Check sheet for the modelled part. Datum: model origin and axes. Units: mm. Round coordinates to 2 decimals unless told otherwise and drop trailing zeros. Loops run counter-clockwise (first coordinate to the right, second up) from the corner with the lowest first, then second, coordinate; pieces in that order, holes last. Notation, with made-up numbers: (67, -18) - (98, -18) arc R33 ccw to (98, 13) - close; hole circle Ø1 at (19, 59). An arc over 180 degrees is marked (long way). Answer in a Markdown table with one row per item. Add a question column.
(1) Cross-section at A-A on z = -84. Enter the section's corners in (x, y), then the cut area to 3 significant figures.
(2) Thickness scan on line 1 along Y through (x, z) = (0, -12); line 2 along X through (y, z) = (23, -155.5); line 3 along Y through (x, z) = (326, -58.5). Record the ranges inside material, lowest first.
(3) Gauge pin test, flat ends, axial feed: pin 1 (12 mm diameter, centred on x = -119.5, y = 486, fed in from +Z); pin 2 (3 mm diameter, centred on x = -34.5, y = -123.5, fed in from +Z); pin 3 (3 mm diameter, centred on y = -103, z = -74, fed in from +X). Record the tip position at first contact, or that the pin passes through.
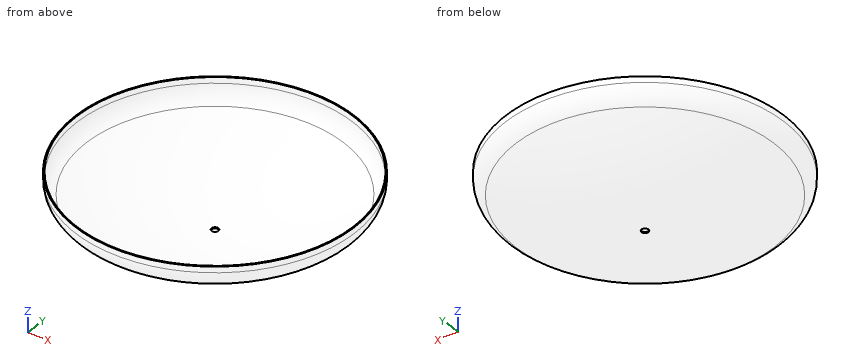
Autodesk Inventor part; units mm, degrees
ref_plane "YZ Plane" through (0, 0, 0) normal (1, 0, 0) x (0, 1, 0)
ref_plane "XZ Plane" through (0, 0, 0) normal (0, 1, 0) x (-1, 0, 0)
ref_plane "XY Plane" through (0, 0, 0) normal (0, 0, 1) x (1, 0, 0)
sketch "Sketch1" plane through (0, 0, 0) normal (0, 1, 0) x (-1, 0, 0)
  line L0 (700, 0) -> (700, -30)
  arc A0 (649.8242, -116.7038) -> (700, -30) centre (600, -30) ccw
  arc A1 (17.5, -290) -> (649.8242, -116.7038) centre (0, 1014.1164) ccw
  line L1 (0, 290) -> (0, -290)
  arc A2 (17.5, -283.9995) -> (646.8348, -111.5016) centre (0, 1014.1164) ccw
  arc A3 (646.8348, -111.5016) -> (694, -30) centre (600, -30) ccw
  line L2 (694, -30) -> (694, 0)
  line L3 (694, 0) -> (700, 0)
  line L4 (0, -290) -> (17.5, -290)
  line L5 (0, -283.9995) -> (17.5, -283.9995)
  line L6 (17.5, -290) -> (17.5, -283.9995)
  point P0 (0, 0)
  point P1 (0, 0)
  point P2 (0, -163.7009)
  point P3 (0, -169.7009)
  dimension "d0" = 100
  dimension "d1" = 30
  dimension "d3" = 1304.2338
  dimension "d6" = 6
  dimension "d13" = 35
  dimension "d14" = 1400
  dimension "d15" = 290
revolve "Revolution1" add sketch "Sketch1" angle 360 about axis through (0, 0, 290) along (0, 0, -1) contours L0 A0 A1 L6 A2 A3 L2 L3
equation "\"d0\" = tech_dishhead_small_rad"
equation "\"d1\" = tech_dishhead_edge_hight"
equation "\"d13\" = tech_dishhead_bottom_hole"
equation "\"d14\" = MAIN_filter_diam"
properties part number "APN 1408 dished head" material "Steel"
Answers:
| question | item | result |
|---|---|---|
| 1 | outline | circle Ø1368.33 at (0, 0); hole circle Ø1353.88 at (0, 0) |
| 1 | area | 30,900 mm^2 |
| 2 | line 1 | y = -700 to -694, 694 to 700 |
| 2 | line 2 | x = -576.62 to -562.92, 562.92 to 576.62 |
| 2 | line 3 | y = -614.76 to -607.65, 607.65 to 614.76 |
| 3 | pin 1 | stops at z = -181.25 |
| 3 | pin 2 | stops at z = -277.62 |
| 3 | pin 3 | stops at x = 682.83 |
